Answer from the drawing. Dimensions are ordinates in mm from the lowest x, y and z of the part. A direction names the side the tool comes from. Round coordinates to 2 decimals unless told otherwise and drop trailing zeros. Loops run counter-clockwise (first coordinate to the right, second up) from the corner with the lowest first, then second, coordinate; pieces in that order, holes last.
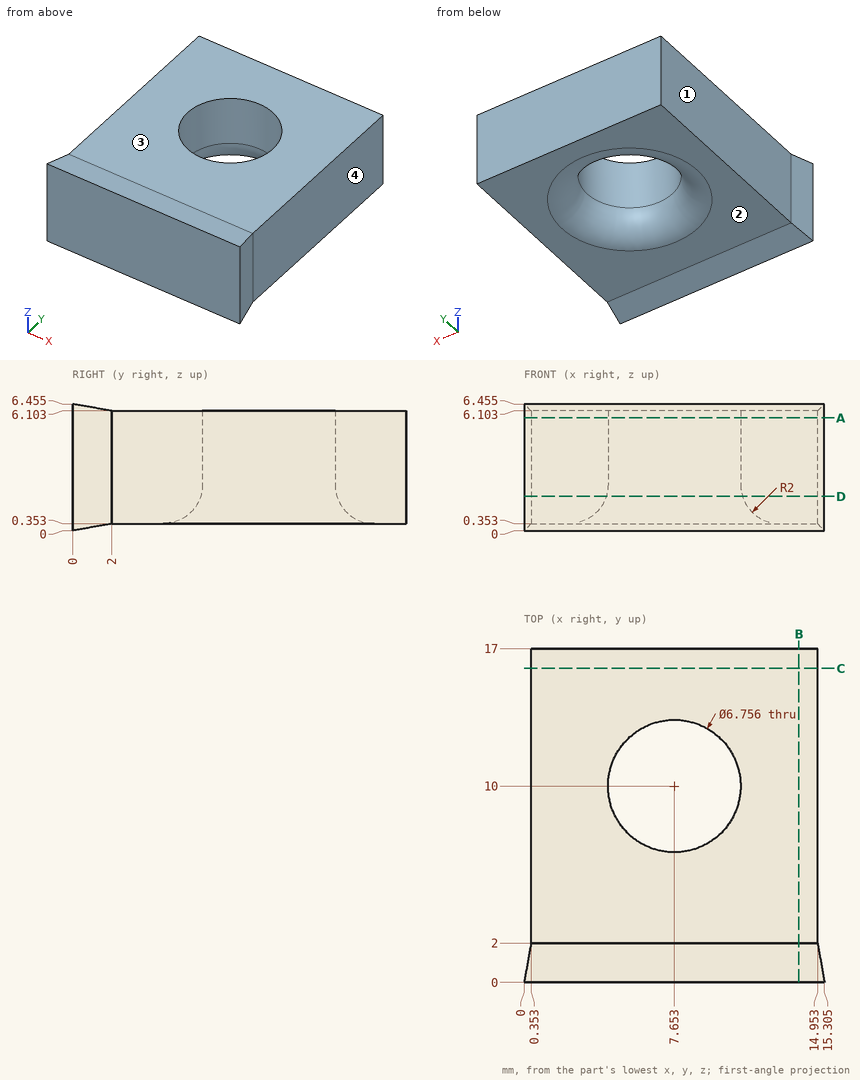
1. Find section A-A (z = 5.75). Write down the section's boundary in (x, y) (1 decimal).
Answer key:
outline: (0, 0) - (15.3, 0) - (15, 2) - (15, 17) - (0.4, 17) - (0.4, 2) - close; hole circle Ø6.8 at (7.7, 10)
2. Find section B-B (x = 14). Write down the section's boundary in (y, z) (1 decimal).
Answer key:
outline: (0, 0) - (2, 0.4) - (17, 0.4) - (17, 6.1) - (2, 6.1) - (0, 6.5) - close
3. Which of the six approach directions +Z, -Z, +X, -X, +Y, -Y give full straight-line access (tool end or side, diameter ignored) to the marked faces 1, 2, 3 and 4?
Answer key:
face 1: +Z, -Z, -X, +Y
face 2: -Z, +X, -X, +Y
face 3: +Z, +X, -X, +Y
face 4: +Z, -Z, +X, +Y
4. Find section C-C (y = 16). Write down the section's boundary in (x, z).
Answer key:
outline: (0.35, 0.35) - (14.95, 0.35) - (14.95, 6.1) - (0.35, 6.1) - close
5. Consider probe 1 along X at (y, z) = (10, 3.7) (1 decimal); probe 2 along Y at (x, z) = (7.5, 4.25) (1 decimal); probe 3 along Z at (x, y) = (14.75, 13.75). Determine where each line is inside the solid, lowest interval first.
Answer key:
probe 1: x = 0.4 to 4.3, 11 to 15
probe 2: y = 0 to 6.6, 13.4 to 17
probe 3: z = 0.35 to 6.1
6. Given pin 1 (7.5 mm diameter, centred on x = 9.5, y = 8, fed in from +Z); pin 2 (5 mm diameter, centred on x = 5.5, y = 2.5, fed in from +Z) (1 decimal); pin 3 (4.5 mm diameter, centred on x = 6.5, y = 7, fed in from -Z); pin 4 (5.5 mm diameter, centred on x = 7.65, y = 10, fed in from +Z), each flat-ended and moving along its own axis, determine where each tip first touches the part or whether it passes through.
Answer key:
pin 1: stops at z = 6.1
pin 2: stops at z = 6.5
pin 3: stops at z = 0.35
pin 4: passes through
7. Find section D-D (z = 1.75). Write down the section's boundary in (x, y) (1 decimal).
Answer key:
outline: (0, 0) - (15.3, 0) - (15, 2) - (15, 17) - (0.4, 17) - (0.4, 2) - close; hole circle Ø6.9 at (7.7, 10)
